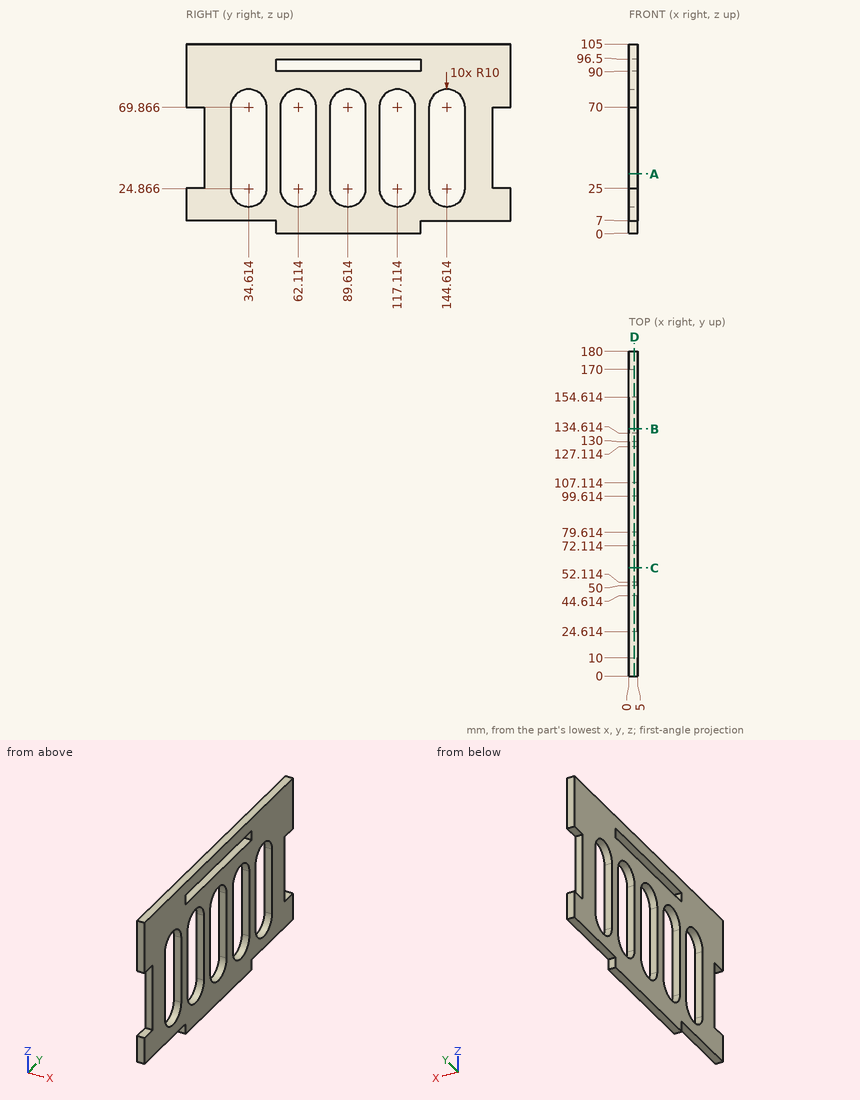
Source: three-view drawing plus pictorial views. Frame: mm from the lowest corner of the part. Give positions to 0.01 mm unless a question says otherwise; leave off trailing zeros. Order: outer loops, then holes, each group sorted by start corner. A loop starts at its lowest first (then second) coordinate and runs counter-clockwise, first axis right, second up. Notation, with made-up numbers: (45.5, 55) -> (104.5, 55) arc R17 ccw to (104.5, 65) -> close; hole circle Ø9 at (0, 15). An arc over 180 degrees is marked (long way). Use a Markdown table: item, result.
Q1. First-contact query: P1, Ø1.5, axis at x = 1, y = 140, coming from the -Z side; P2, Ø1, axis at x = 0.5, z = 66, coming from the -Y side; P3, Ø2, axis at x = 1.5, z = 52.5, coming from the +Y side. Flat tips, straight axial feed; report the tip coordinate or a pass-through.
A:
| item | result |
|---|---|
| P1 | z = 7 |
| P2 | y = 10 |
| P3 | y = 170 |
Q2. Section C-C (y = 60). Return the cut outline in (x, z).
A:
| item | result |
|---|---|
| outline | (0, 0) -> (5, 0) -> (5, 15.09) -> (0, 15.09) -> close; (0, 79.64) -> (5, 79.64) -> (5, 90) -> (0, 90) -> close; (0, 96.5) -> (5, 96.5) -> (5, 105) -> (0, 105) -> close |
Q3. Section B-B (y = 137). Return the cut outline in (x, z).
A:
| item | result |
|---|---|
| outline | (0, 7) -> (5, 7) -> (5, 18.38) -> (0, 18.38) -> close; (0, 76.35) -> (5, 76.35) -> (5, 105) -> (0, 105) -> close |
Q4. Section A-A (z = 33). Return the cut outline in (x, y).
A:
| item | result |
|---|---|
| outline | (0, 10) -> (5, 10) -> (5, 24.61) -> (0, 24.61) -> close; (0, 44.61) -> (5, 44.61) -> (5, 52.11) -> (0, 52.11) -> close; (0, 72.11) -> (5, 72.11) -> (5, 79.61) -> (0, 79.61) -> close; (0, 99.61) -> (5, 99.61) -> (5, 107.11) -> (0, 107.11) -> close; (0, 127.11) -> (5, 127.11) -> (5, 134.61) -> (0, 134.61) -> close; (0, 154.61) -> (5, 154.61) -> (5, 170) -> (0, 170) -> close |
Q5. Material intervals for line 1 (Y direction, x = 3.65, z = 69.5); line 2 (Y direction, x = 3.55, z = 92.5); line 3 (Z direction, x = 0.45, y = 62) (1 decimal), sorted ascending. Write a range as [from, to].
A:
| item | result |
|---|---|
| line 1 | [10, 24.61], [44.61, 52.11], [72.11, 79.61], [99.61, 107.11], [127.11, 134.61], [154.61, 170] |
| line 2 | [0, 50], [130, 180] |
| line 3 | [0, 14.9], [79.9, 90], [96.5, 105] |
Q6. Section D-D (x = 3.1). State how many separate pieces and enclosed holes the cut face has, and give its area (3 significant figures).
A:
| item | result |
|---|---|
| separate pieces | 1 |
| enclosed holes | 6 |
| area | 10,700 mm^2 |
